Answer from the drawing. Dimensions are ordinates in mm from the lowest x, y and z of the part. A direction names the side the tool comes from. Give positions to 0.01 mm unless a question says otherwise; leave off trailing zeros. Write each loop counter-clockwise with the first axis right and the second up, starting at its lowest first coordinate (ties: lowest second). Pieces come first, ordered by that corner, then holes. Notation, with made-up numbers: (-38.75, -32.75) -> (19.25, -32.75) arc R12 cw to (19.25, -22.75) -> close; hole circle Ø8 at (49, 28.25). An arc over 180 degrees is marked (long way). Use a Markdown table: item, result. Add a question column.
Q1. For a pull along Z with two mould halves and no side action, classify the marked faces 3, 4 and 5 as pulls with the +Z half, pulls with the -Z half, needs draft (parallel to the pull), parting line crosses it, or undercut.
Q2. Section A-A, the plane z = 27.88 is taken. Give the vertices of the cut face in (x, y) (1 decimal), plus the area to 3 significant figures.
Q3. For the marked faces 1 and 2, determine the directions among +Z, -Z, +X, -X, +Y, -Y from which every point of the face is accessible in a straight line to the end or side of a thin tool.
Q4. Each of these flat-tipped pins is pushed along its axis until it touches: pin 1 Ø1 at (y, z) = (20, 20) entering from +X; pin 2 Ø9 at (x, y) = (10, 17) entering from +Z. Where does it stop, or does it pass through?
Q5. Consider line 1 (Y direction, x = 1.5, z = 12); line 2 (Y direction, x = 16.75, z = 27); line 3 (X direction, y = 13, z = 19). Determine where each line is inside the solid, lowest interval first.
Q6. Section B-B, the plane y = 49.6 is taken. Give the vertices of the cut face in (x, z) (1 decimal).
Q7. Section C-C, the plane x = 10.75 is taken. Give the vertices of the cut face in (y, z).
Q8. Section D-D, the plane z = 7 is taken. Give the vertices of the cut face in (x, y), plus the area to 3 significant figures.
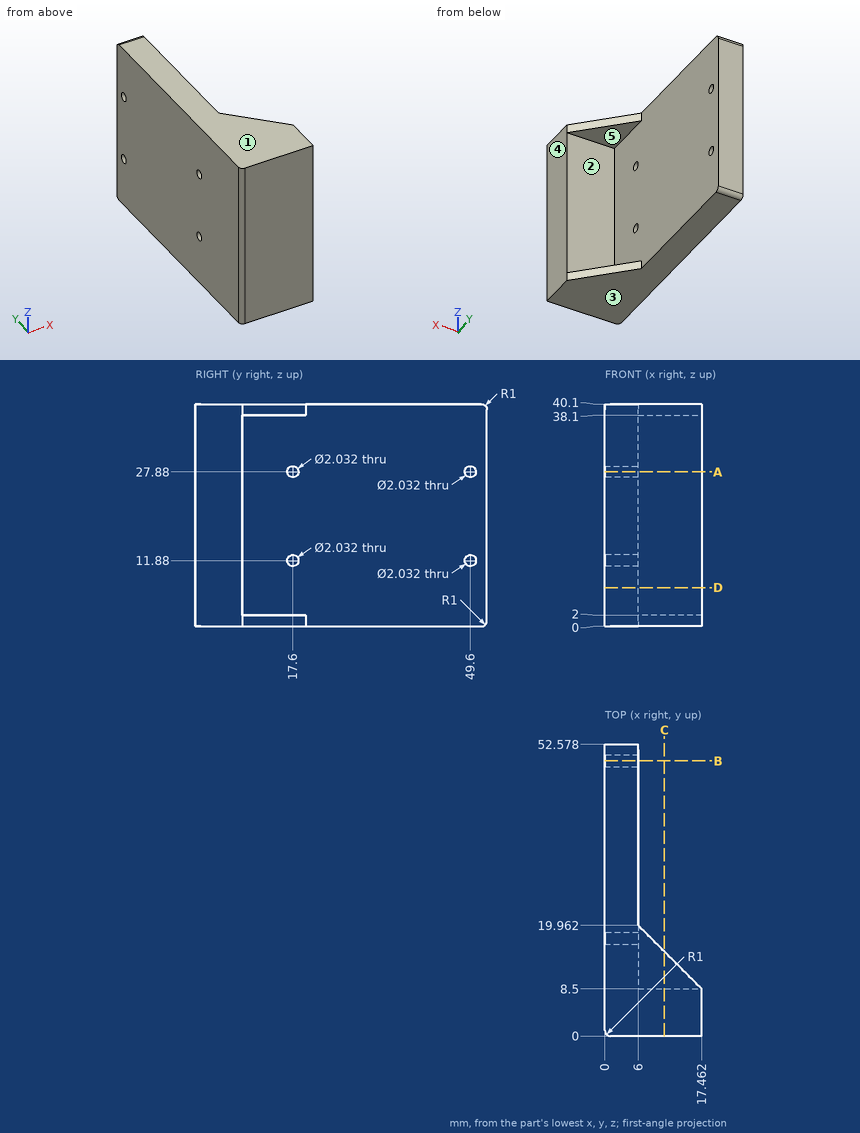
Result set:
| question | item | result |
|---|---|---|
| 1 | face 3 | pulls with the -Z half |
| 1 | face 4 | needs draft |
| 1 | face 5 | undercut |
| 2 | outline | (0, 1) arc R1 ccw to (1, 0) -> (17.5, 0) -> (17.5, 8.5) -> (6, 8.5) -> (6, 16.6) -> (0, 16.6) -> close; (0, 18.6) -> (6, 18.6) -> (6, 48.6) -> (0, 48.6) -> close; (0, 50.6) -> (6, 50.6) -> (6, 52.6) -> (0, 52.6) -> close |
| 2 | area | 388 mm2 |
| 3 | face 1 | +Z, +X, -X, +Y, -Y |
| 3 | face 2 | +X, +Y |
| 4 | pin 1 | stops at x = 6 |
| 4 | pin 2 | stops at z = 40.1 |
| 5 | line 1 | y = 0 to 16.59, 18.61 to 48.59, 50.61 to 52.58 |
| 5 | line 2 | y = 0 to 8.5 |
| 5 | line 3 | x = 0 to 6 |
| 6 | outline | (0, 0) -> (6, 0) -> (6, 10.9) -> (0, 10.9) -> close; (0, 12.9) -> (6, 12.9) -> (6, 26.9) -> (0, 26.9) -> close; (0, 28.9) -> (6, 28.9) -> (6, 40.1) -> (0, 40.1) -> close |
| 7 | outline | (0, 0) -> (15.21, 0) -> (15.21, 2) -> (8.5, 2) -> (8.5, 38.1) -> (15.21, 38.1) -> (15.21, 40.1) -> (0, 40.1) -> close |
| 8 | outline | (0, 1) arc R1 ccw to (1, 0) -> (17.46, 0) -> (17.46, 8.5) -> (6, 8.5) -> (6, 52.58) -> (0, 52.58) -> close |
| 8 | area | 413 mm2 |
